```python
from build123d import *

# Parameters (mm, degrees)
SKETCH1_W           = 138.92560988
SKETCH1_H           = 12.7
SKETCH1_R           = 1.778
BOSS_EXTRUDE1_DEPTH = 3.175
SKETCH2_W           = 3.175
SKETCH2_H           = 12.7
BOSS_EXTRUDE2_DEPTH = 63.5
SKETCH3_R           = 1.778
CUT_EXTRUDE1_DEPTH  = 152.4
BOSS_EXTRUDE3_REACH = 156.619
BOSS_EXTRUDE4_DEPTH = 63.5
FILLET1_R           = 6.35


with BuildPart() as part:
    # Sketch1 → Boss-Extrude1 (new body)
    with BuildSketch(Plane.XY):
        with Locations((-69.46280494, -6.35)):
            Rectangle(SKETCH1_W, SKETCH1_H)
        with Locations((-94.86280494, -6.35)):
            Circle(SKETCH1_R, mode=Mode.SUBTRACT)
        with Locations((-44.06280494, -6.35)):
            Circle(SKETCH1_R, mode=Mode.SUBTRACT)
    extrude(amount=BOSS_EXTRUDE1_DEPTH)

    # Sketch2 → Boss-Extrude2 (add)
    with BuildSketch(Plane.XY.offset(3.175)):
        with Locations((-137.33810988, -6.35)):
            Rectangle(SKETCH2_W, SKETCH2_H)
        with Locations((-1.5875, -6.35)):
            Rectangle(SKETCH2_W, SKETCH2_H)
    extrude(amount=BOSS_EXTRUDE2_DEPTH)

    # Sketch3 → Cut-Extrude1 (cut)
    with BuildSketch(Plane(origin=(0, 0, 0), x_dir=(0, 0, -1), z_dir=(1, 0, 0))):
        with Locations(Location((-56.840236332, -6.35, 0), (0, 0, 90))):
            Circle(SKETCH3_R)
    extrude(amount=-CUT_EXTRUDE1_DEPTH, mode=Mode.SUBTRACT)

    # Boss-Extrude3: up to this face of the body (flat: up to its plane)
    boss_extrude3_end = Plane(part.part.faces().sort_by_distance((-138.92560988, -6.35, 33.058574097))[0])
    # Sketch5 → Boss-Extrude3 (add, up to the picked face)
    with BuildSketch(Plane(origin=(0, 0, 0), x_dir=(0, 0, -1), z_dir=(1, 0, 0)), mode=Mode.PRIVATE) as boss_extrude3_sk1:
        Polygon((-3.175, 0), (13.49375, 28.871121899), (15.875, 27.49630657), (0, 0), align=None)
    boss_extrude3_tool1 = split(extrude(boss_extrude3_sk1.sketch, amount=-BOSS_EXTRUDE3_REACH, mode=Mode.PRIVATE), bisect_by=boss_extrude3_end, keep=Keep.BOTH, mode=Mode.PRIVATE)
    add(boss_extrude3_tool1.solids().sort_by(Axis((0, 14.094651, -6.537144), (-1, 0, 0)))[0])

    # Sketch6 → Boss-Extrude4 (add)
    with BuildSketch(Plane.XY.offset(66.675)):
        Polygon((-3.175, 0), (13.513581363, 28.905470827), (16.241711333, 27.281299694), (0, 0), align=None)
        Polygon((-138.92560988, 0), (-155.167321213, 27.281299694), (-152.439191243, 28.905470827), (-135.75060988, 0), align=None)
    extrude(amount=-BOSS_EXTRUDE4_DEPTH)

    # Fillet1
    fillet1_edges = [part.edges().sort_by_distance(p)[0] for p in [
        (-69.46280494, 0, 0),
        (-138.92560988, 0, 34.925),
        (0, 0, 34.925),
    ]]
    fillet(fillet1_edges, radius=FILLET1_R)


solid = part.part
```
Input: part model. Units: mm. Frame: model coordinates. A direction names the side the tool comes from. Give positions to 0.01 mm unless a question says otherwise; leave off trailing zeros. Order: outer loops, then holes, each group sorted by start corner. A loop starts at its lowest first (then second) coordinate and runs counter-clockwise, first axis right, second up. Notation, with made-up numbers: (0, 66.5) - (29, 66.5) arc R17 cw to (29, 71.5) - close; hole circle Ø11 at (-11, 20). An arc over 180 degrees is marked (long way). One line per item, written item: value.
1. Pin query (flat end, axial travel): pin 1 Ø1 at (x, z) = (-112, -1) entering from -Y; pin 2 Ø2 at (x, z) = (-137, -7) entering from +Y; pin 3 Ø21 at (y, z) = (-1.5, 41.5) entering from -X. Return the tip coordinate at first contact, or that it passes through.
Determined:
pin 1: y = 0.77
pin 2: y = 19.36
pin 3: x = -144.28
2. Cut plane D-D, the plane x = -36.5. Output: boundary loops of the cut face in (y, z) (3 decimals), and give its area (3 significant figures).
Determined:
outline: (-12.7, 0) - (-1.701, 0) arc R6.35 cw to (1.474, -0.851) - (27.496, -15.875) - (28.871, -13.494) - (0, 3.175) - (-12.7, 3.175) - close
area: 130 mm2
3. Cut plane C-C, the plane y = 17. Output: boundary loops of the cut face in (x, z) (3 decimals).
Determined:
outline: (-149.046, 3.175) - (-145.566, 3.175) - (-145.566, 66.675) - (-149.046, 66.675) - close; (-138.926, -9.815) - (0, -9.815) - (0, -6.64) - (-138.926, -6.64) - close; (6.64, 3.175) - (10.121, 3.175) - (10.121, 66.675) - (6.64, 66.675) - close
4. Cut plane A-A, the plane y = -6.35. Output: boundary loops of the cut face in (x, z) (3 decimals), and give its area (3 significant figures).
Determined:
outline: (-138.926, 0) - (-96.641, 0) - (-96.641, 3.175) - (-135.751, 3.175) - (-135.751, 55.062) - (-138.926, 55.062) - close; (-138.926, 58.618) - (-135.751, 58.618) - (-135.751, 66.675) - (-138.926, 66.675) - close; (-93.085, 0) - (-45.841, 0) - (-45.841, 3.175) - (-93.085, 3.175) - close; (-42.285, 0) - (0, 0) - (0, 55.062) - (-3.175, 55.062) - (-3.175, 3.175) - (-42.285, 3.175) - close; (-3.175, 58.618) - (0, 58.618) - (0, 66.675) - (-3.175, 66.675) - close
area: 799 mm2
5. Reachability of faces 5 (the face through (-3.175, -6, 34)), 6 (the face through (-139.147, -0.086, 34.48)), 7 (the face through (5.05, 14.25, 35.37)) from +Z, -Z, +X, -X, +Y, -Y: full face, straight path, thin tool, end or side. Return the list, or none.
Determined:
face 5: +Z, +Y, -Y
face 6: +Z, -Z, -X, -Y
face 7: +Z, +Y
6. Cut plane B-B, the plane z = 35.5. Output: boundary loops of the cut face in (x, y) (3 decimals), and give its area (3 significant figures).
Determined:
outline: (-155.167, 27.281) - (-139.819, 1.501) arc R6.35 cw to (-138.926, -1.747) - (-138.926, -12.7) - (-135.751, -12.7) - (-135.751, 0) - (-152.439, 28.905) - close; (-3.175, -12.7) - (0, -12.7) - (0, -1.747) arc R6.35 cw to (0.894, 1.501) - (16.242, 27.281) - (13.514, 28.905) - (-3.175, 0) - close
area: 274 mm2
7. Line query: probe 1 along Z at (x, y) = (-137, -6) (3 decimals); probe 2 along Z at (x, y) = (-107, -5) (3 decimals); probe 3 along X at (y, z) = (-3.5, 61) (3 decimals). Output: solid intervals per line, ascending.
Determined:
probe 1: 0 to 55.097, 58.583 to 66.675
probe 2: 0 to 3.175
probe 3: -138.926 to -135.751, -3.175 to 0
8. Draft query along X for faces 1 (the face through (8.675, 14.572, 35.369)), 2 (the face through (-144.212, 14.655, 35.369)), 3 (the face through (-147.386, 14.211, 35.369)), 4 (the face through (-137.3, -7.7, 58)). Return one class per face: released by +X, released by -X, zero draft, split by the parting line, or undercut.
Determined:
face 1: released by +X
face 2: undercut
face 3: released by -X
face 4: zero draft
